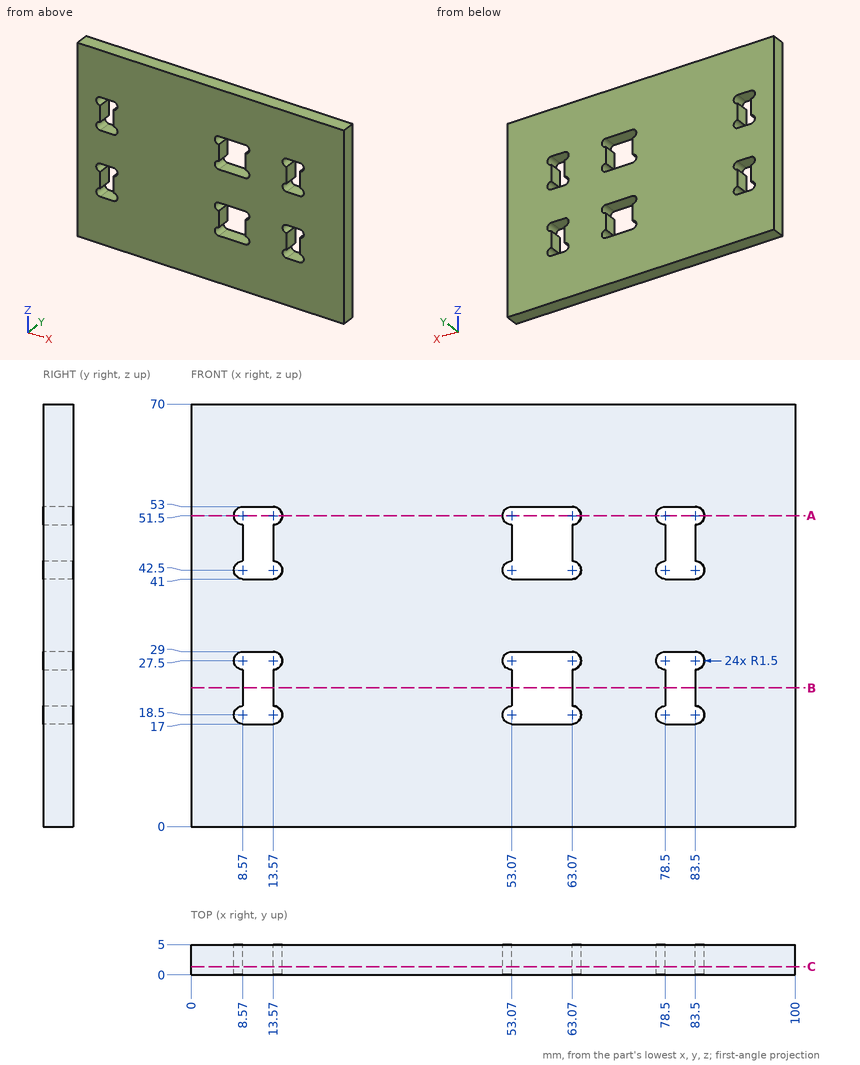
Job drawing, mm, ordinate dimensions from the low corner. One solid piece. Coordinates: 2 decimals unless noted, no trailing zeros. Order: outer loops, then holes, each group sorted by start corner. A loop starts at its lowest first (then second) coordinate and runs counter-clockwise, first axis right, second up. Notation, with made-up numbers: (21.5, -31) - (64.5, -31) arc R31 cw to (64.5, 2) - close; hole circle Ø8 at (50.5, 28.25). An arc over 180 degrees is marked (long way). Return JSON: item names as keys, results as strings. Group by question number.
1) Saw through at A-A, the plane z = 51.5. Write the cut outline in (x, y), plus the area to 3 significant figures.
2) Probe line 1 (X direction, y = 2.7, z = 21); line 2 (Z direction, x = 54.5, y = 4.4); line 3 (X direction, y = 1.65, z = 51.5). List the from-to ranges inside material, lowest first. Write a range as from..to.
3) Saw through at C-C, the plane y = 1.35. Count the separate pieces of the cut face and the enclosed holes in it, plus the area to 3 significant figures.
4) Saw through at B-B, the plane z = 23. Write the cut outline in (x, y).
Values found:
{
 "1": {"outline": "(0, 0) - (7.07, 0) - (7.07, 5) - (0, 5) - close; (15.07, 0) - (51.57, 0) - (51.57, 5) - (15.07, 5) - close; (64.57, 0) - (77, 0) - (77, 5) - (64.57, 5) - close; (85, 0) - (100, 0) - (100, 5) - (85, 5) - close", "area": "355 mm²"},
 "2": {"line 1": "x = 0..8.57, 13.57..53.07, 63.07..78.5, 83.5..100", "line 2": "z = 0..17, 29..41, 53..70", "line 3": "x = 0..7.07, 15.07..51.57, 64.57..77, 85..100"},
 "3": {"separate pieces": "1", "enclosed holes": "6", "area": "6,440 mm²"},
 "4": {"outline": "(0, 0) - (8.57, 0) - (8.57, 5) - (0, 5) - close; (13.57, 0) - (53.07, 0) - (53.07, 5) - (13.57, 5) - close; (63.07, 0) - (78.5, 0) - (78.5, 5) - (63.07, 5) - close; (83.5, 0) - (100, 0) - (100, 5) - (83.5, 5) - close"}
}
